from build123d import *

# Parameters (mm, degrees)
F0_R     = 4.74599
F1_DEPTH = 152.4
F3_DEPTH = 8.334375
F4_R     = 1.27


# Not quite as in the source:
# - a length typed as a fraction of an inch, garbled in the dataset ("3 / 203.2 mm" for 3/8 in), is restored


with BuildPart() as f1:
    # F0 (on Top) → F1 (new body)
    with BuildSketch(Plane.XY):
        Circle(F0_R)
    extrude(amount=F1_DEPTH)

    # F2 (on Top) → F3 (join)
    with BuildSketch(Plane.XY):
        Polygon((-4.1244459855, -7.14375), (4.1244459855, -7.14375), (8.248891971, 0), (4.1244459855, 7.14375), (-4.1244459855, 7.14375), (-8.248891971, 0), align=None)
    extrude(amount=F3_DEPTH)

    # F4
    f4_edges = [f1.edges().sort_by_distance(p)[0] for p in [
        (-4.74599, 0, 152.4),
    ]]
    fillet(f4_edges, radius=F4_R)


solid = f1.part
For this review, take the finished solid that the model builds, in its own axes (mm). A direction names the side the tool comes from. Round coordinates to 2 decimals unless told otherwise and drop trailing zeros. Order: outer loops, then holes, each group sorted by start corner. A loop starts at its lowest first (then second) coordinate and runs counter-clockwise, first axis right, second up. Notation, with made-up numbers: (-28, 80) -> (6, 80) arc R13 cw to (6, 87) -> close; hole circle Ø3 at (9, 9.25). An arc over 180 degrees is marked (long way). Write item = value, one per line. Start each with the question number.
1) Tool access review of faces 1 (the face through (6.16, -3.62, 4.11)), 2 (the face through (-3.766, -2.888, 78.733)): name each direction out of +Z, -Z, +X, -X, +Y, -Y from which nothing blocks a thin tool from reaching the whole face with its end or side.
2) Insertion check: pin 1 (5 mm diameter, centred on y = 0, z = 108, fed in from -X); pin 2 (8 mm diameter, centred on y = -4, z = 124.5, fed in from +X); pin 3 (8 mm diameter, centred on x = -6, z = 77.5, fed in from +Y). Each pin has a flat end and moves straight along its axis. Give the tip position at first contact, or say it passes through.
3) Take a section at C-C on x = 6.5. State the section outline as (y, z) points.
4) Take a section at A-A on x = 0. State the section outline as (y, z) points, plus the area to 3 significant figures.
5) To check wall thickness, follow line 1 (Z direction, x = -4.5, y = -4.25); line 2 (X direction, y = 3.25, z = 138); line 3 (X direction, y = -0.25, z = 143). State the ranges of each line that lie inside material, in increasing order. Write a range as from..to.
6) Take a section at B-B on z = 29.5. State the section outline as (x, y) points.
Verdict:
q1.face_1 = +Z, -Z, +X, -Y
q1.face_2 = +Z
q2.pin_1 = -4.75
q2.pin_2 = 4.75
q2.pin_3 = 4.3
q3.outline = (-3.03, 0) -> (3.03, 0) -> (3.03, 8.33) -> (-3.03, 8.33) -> close
q4.outline = (-7.14, 0) -> (7.14, 0) -> (7.14, 8.33) -> (4.75, 8.33) -> (4.75, 151.13) arc R1.27 ccw to (3.48, 152.4) -> (-3.48, 152.4) arc R1.27 ccw to (-4.75, 151.13) -> (-4.75, 8.33) -> (-7.14, 8.33) -> close
q4.area = 1,490 mm2
q5.line_1 = 0..8.33
q5.line_2 = -3.46..3.46
q5.line_3 = -4.74..4.74
q6.outline = circle Ø9.49 at (0, 0)
